The listing builds one solid part. Answer for the finished solid, in the listing's coordinates (mm). Face numbers are marked on the shaded views. A direction names the side the tool comes from. Coordinates: 2 decimals unless noted, no trailing zeros. Loops run counter-clockwise (first coordinate to the right, second up) from the corner with the lowest first, then second, coordinate; pieces in that order, holes last. Notation, with made-up numbers: (-21, 45.5) - (-5, 45.5) arc R21 ccw to (-5, 55.5) - close; hole circle Ø6 at (56, 11). An arc over 180 degrees is marked (long way). Return JSON: item names as keys, results as strings. Group by question number.
1. The mould has two halves that part along Z. Classify the marked faces 4, 5, 6 and 7: pulls with the +Z half, pulls with the -Z half, needs draft (parallel to the pull), parting line crosses it, or undercut.
2. Section A-A (z = 0) is taken. Write down the section's boundary in (x, y).
3. Each of these flat-tipped pins is pushed along its axis until it touches: P1, Ø1.5, axis at y = 1, z = 30, coming from the +X side; P2, Ø4, axis at x = 66.5, y = -8, coming from the +Z side; P3, Ø4, axis at x = 67, z = -4.5, coming from the -Y side. Where does it stop, or does it pass through?
4. Section B-B (x = 55.5) is taken. Write down the section's boundary in (y, z).
5. Which of the six approach directions +Z, -Z, +X, -X, +Y, -Y give full straight-line access (tool end or side, diameter ignored) to the marked faces 1, 2 and 3?
6. Section C-C (z = -21.5) is taken. State how many separate pieces and enclosed holes the cut face has, and give its area (3 significant figures).
7. Section D-D (x = 23.5) is taken. Write down the section's boundary in (y, z).
8. Find the intervals of material crossed by line 1 along Z through (x, y) = (67.9, -25.25); line 2 along Y through (x, z) = (67, 21); line 3 along Z through (x, y) = (54.75, 0), in increasing order.
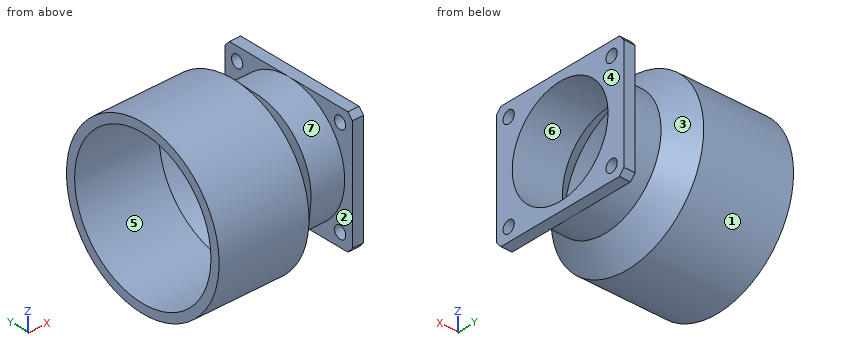
Autodesk Inventor part; units mm, degrees
ref_plane "YZ Plane" through (0, 0, 0) normal (1, 0, 0) x (0, 1, 0)
ref_plane "XZ Plane" through (0, 0, 0) normal (0, 1, 0) x (-1, 0, 0)
ref_plane "XY Plane" through (0, 0, 0) normal (0, 0, 1) x (1, 0, 0)
sketch "Skizze1" plane through (0, 0, 0) normal (0, 0, 1) x (1, 0, 0)
  line L0 (40.05, 37.45) -> (50, 27.5)
  line L1 (50, 27.5) -> (65, 27.5)
  line L2 (65, 27.5) -> (65, 40)
  line L3 (65, 40) -> (70, 40)
  line L4 (70, 40) -> (70, 0)
  line L5 (70, 0) -> (0, 0)
  line L6 (0, 23.5) -> (70, 23.5)
  line L7 (0, 0) -> (0, 37.45)
  line L8 (0, 37.45) -> (40.05, 37.45)
  line L9 (0, 33.45) -> (37.6704, 33.45)
  line L10 (37.6704, 33.45) -> (47.6204, 23.5)
  dimension "d0" = 23.5
  dimension "d2" = 5
  dimension "d3" = 15
  dimension "d6" = 40
  dimension "d7" = 4
  dimension "d34" = 37.45
  dimension "d35" = 135
  dimension "d36" = 70
  dimension "d52" = 4
revolve "Umdrehung2" add sketch "Skizze1" angle 360 about axis through (70, 0, 0) along (-1, 0, 0) contours L0 L1 L2 L3 L4 L6 L10 L9 L7 L8
sketch "Skizze5" plane through (70, 0, 0) normal (1, 0, 0) x (0, 0, -1)
  circle A0 centre (0, 0) radius 40
  line L0 (-27.5, 29.0474) -> (-27.5, -29.0474)
  line L1 (27.5, 29.0474) -> (27.5, -29.0474)
  line L2 (-24.9687, -31.25) -> (24.9687, -31.25)
  line L3 (-24.9687, 31.25) -> (24.9687, 31.25)
  circle A1 centre (0, 0) radius 37.45
  circle A2 centre (0, 0) radius 40
  point P0 (0, 31.25)
  point P1 (-27.5, 0)
  dimension "d38" = 62.5
  dimension "d40" = 55
extrude "Extrusion3" cut sketch "Skizze5" against normal up to surface (5 mm away) contours A0 L1 A1 | L3 A1 A0 | A1 L1 | A0 L2 A1 | L3 A1 | A1 L2 | L0 A1 A0 | L0 A1
sketch "Skizze6" plane through (70, -29.0474, -27.5) normal (1, 0, 0) x (0, 0, -1)
  line L0 (-55, -2.2026) -> (-49, -2.2026)
  line L1 (-49, -2.2026) -> (-49, 3.7974)
  line L2 (-49, 3.7974) -> (-55, 3.7974)
  line L3 (-55, 3.7974) -> (-55, -2.2026)
  line L4 (-55, 60.2974) -> (-49, 60.2974)
  line L5 (-49, 60.2974) -> (-49, 54.2974)
  line L6 (-49, 54.2974) -> (-55, 54.2974)
  line L7 (-55, 54.2974) -> (-55, 60.2974)
  line L8 (0, 60.2974) -> (-6, 60.2974)
  line L9 (-6, 60.2974) -> (-6, 54.2974)
  line L10 (-6, 54.2974) -> (0, 54.2974)
  line L11 (0, 54.2974) -> (0, 60.2974)
  line L12 (0, 3.7974) -> (-6, 3.7974)
  line L13 (-6, 3.7974) -> (-6, -2.2026)
  line L14 (-6, -2.2026) -> (0, -2.2026)
  line L15 (0, -2.2026) -> (0, 3.7974)
  circle A0 centre (-27.5, 29.0474) radius 23.5
  line L16 (0, 0) -> (0, 58.0948)
  arc A1 (0, 58.0948) -> (-2.5313, 60.2974) centre (-27.5, 29.0474) ccw
  line L17 (-2.5313, 60.2974) -> (-52.4687, 60.2974)
  arc A2 (-52.4687, 60.2974) -> (-55, 58.0948) centre (-27.5, 29.0474) ccw
  line L18 (-55, 58.0948) -> (-55, 0)
  arc A3 (-55, 0) -> (-52.4687, -2.2026) centre (-27.5, 29.0474) ccw
  line L19 (-52.4687, -2.2026) -> (-2.5313, -2.2026)
  arc A4 (-2.5313, -2.2026) -> (0, 0) centre (-27.5, 29.0474) ccw
  line L20 (0, 0) -> (0, 58.0948)
  line L21 (-2.5313, 60.2974) -> (-52.4687, 60.2974)
  line L22 (-55, 58.0948) -> (-55, 0)
  line L23 (-52.4687, -2.2026) -> (-2.5313, -2.2026)
  dimension "d43" = 6
hole "Bohrung2" at (70, -25.25, 21.5) at (70, 25.25, 21.5) at (70, 25.25, -21.5) at (70, -25.25, -21.5) direction (-1, 0, 0) diameter 5.5 depth 8 tip angle 118
properties part number "Rohrhalterung_2"
The answers:
{
 "1": {"face 4": "needs draft", "face 5": "undercut", "face 6": "undercut", "face 7": "parting line crosses it"},
 "2": {"outline": "(0, -37.45) - (40.05, -37.45) - (50, -27.5) - (65, -27.5) - (65, -31.25) - (70, -31.25) - (70, -23.5) - (47.62, -23.5) - (37.67, -33.45) - (0, -33.45) - close; (0, 33.45) - (37.67, 33.45) - (47.62, 23.5) - (70, 23.5) - (70, 31.25) - (65, 31.25) - (65, 27.5) - (50, 27.5) - (40.05, 37.45) - (0, 37.45) - close"},
 "3": {"P1": "stops at x = 48.23", "P2": "stops at z = 27.5", "P3": "stops at y = -31.25"},
 "4": {"outline": "circle Ø55 at (0, 0); hole circle Ø47 at (0, 0)"},
 "5": {"face 1": "-X", "face 2": "-Y", "face 3": "none"},
 "6": {"separate pieces": "4", "enclosed holes": "0", "area": "989 mm2"},
 "7": {"outline": "circle Ø74.9 at (0, 0); hole circle Ø66.9 at (0, 0)"},
 "8": {"line 1": "z = -27.5 to -24.25, -18.75 to 18.75, 24.25 to 27.5", "line 2": "y = -31.25 to -27.95, -22.55 to -10.55, 10.55 to 22.55, 27.95 to 31.25", "line 3": "z = -27.5 to -23.5, 23.5 to 27.5"}
}
